For this review, take the finished solid that the model builds, in its own axes (mm). Face numbers are marked on the shaded views. A direction names the side the tool comes from. Coordinates: 2 decimals unless noted, no trailing zeros. Order: outer loops, then holes, each group sorted by start corner. A loop starts at its lowest first (then second) coordinate and runs counter-clockwise, first axis right, second up. Notation, with made-up numbers: (-12.5, 0.5) -> (41.5, 0.5) arc R30 cw to (41.5, 31.5) -> close; hole circle Ø9 at (-1.5, 63.25). An arc over 180 degrees is marked (long way). Answer as a JSON object with one key per item and string values. Group by question number.
1) For pin 1 (8 mm diameter, centred on x = -6, z = -4.5, fed in from -Y); pin 2 (2 mm diameter, centred on x = -7.5, y = 3, fed in from +Z); pin 3 (1 mm diameter, centred on x = -3.5, y = 3.5, fed in from +Z); pin 4 (5.5 mm diameter, centred on x = -10.5, z = 0, fed in from +Y), all flat-tipped, find the tip position at first contact; note any pin that passes through.
2) Add section C-C, the plane y = 0.7. Write out the cut boundary in (x, z), then the cut area to 3 significant figures.
3) Add section A-A, the plane x = -10.5. Write out the cut boundary in (y, z), then the cut area to 3 significant figures.
4) Machinability: for the marked faces 4, 5 and 6, which of the approach directions +Z, -Z, +X, -X, +Y, -Y give a long, thin tool a straight path to every point of the face, cutting with its end or side? Answer none if there is none.
5) Add section D-D, the plane x = -5.25. Write out the cut boundary in (y, z).
6) Wall thickness on L1, parallel to X at y = 0.7, z = 0; L2, parallel to Z at x = -10.5, y = 0.85; L3, parallel to X at y = 0.45, z = -1.5: over which ranges is each line inside the solid? List them lowest first.
7) Draft analysis for pull direction X (two halves, no side actions). For the marked faces 1, 2 and 3, state which applies: +X half, -X half, draft (parallel to the pull), parting line (faces both ways), or undercut.
Autodesk Inventor part; units mm, degrees
ref_plane "YZ Plane" through (0, 0, 0) normal (1, 0, 0) x (0, 1, 0)
ref_plane "XZ Plane" through (0, 0, 0) normal (0, 1, 0) x (-1, 0, 0)
ref_plane "XY Plane" through (0, 0, 0) normal (0, 0, 1) x (1, 0, 0)
sketch "Szkic1" plane through (0, 0, 0) normal (0, 1, 0) x (-1, 0, 0)
  line L0 (-15, 8) -> (15, 8)
  line L1 (15, 8) -> (15, -8)
  line L2 (15, -8) -> (-15, -8)
  line L3 (-15, -8) -> (-15, 8)
  line L4 (-15, 8) -> (15, -8) construction
  line L5 (15, 8) -> (-15, -8) construction
  line L6 (-6, 6) -> (6, 6)
  line L7 (6, 6) -> (6, -6)
  line L8 (6, -6) -> (-6, -6)
  line L9 (-6, -6) -> (-6, 6)
  line L10 (-6, 6) -> (6, -6) construction
  line L11 (6, 6) -> (-6, -6) construction
  circle A0 centre (0, 0) radius 1.75
  dimension "d0" = 30
  dimension "d1" = 16
  dimension "d2" = 12
  dimension "d3" = 12
  dimension "d4" = 3.5
extrude "Wyciągnięcie proste1" add sketch "Szkic1" along normal blind 1.4 contours L0 L1 L2 L3 | L6 L7 L8 L9 | A0
extrude "Wyciągnięcie proste2" add sketch "Szkic1" along normal blind 1.6 contours L6 L7 L8 L9 | A0
extrude "Wyciągnięcie proste3" cut sketch "Szkic1" along normal blind 1 contours A0
chamfer "Faza1" distance 4 angle 45 4 edges at (15, 0.7, 8) (15, 0.7, -8) (-15, 0.7, 8) (-15, 0.7, -8)
offset faces "Rozmiar1" outward -0.5 faces at (-3.6667, 0.4667, 8) (-12.3333, 0.4667, 6.6667) (12.3333, 0.4667, 6.6667) (15, 0.4667, 1.3333) (13.6667, 0.4667, -5.3333) (3.6667, 0.4667, -8) (-13.6667, 0.4667, -5.3333) (-15, 0.4667, -1.3333)
sketch "Szkic2" plane through (0, 1.4, 0) normal (0, 1, 0) x (1, 0, 0)
  line L0 (-6, -6) -> (6, -6)
  line L1 (-6, 6) -> (6, 6)
  line L2 (-6, -6) -> (6, -6)
  line L3 (6, -6) -> (6, 6)
  line L4 (6, 6) -> (-6, 6)
  line L5 (-6, 6) -> (-6, -6)
  line L6 (0, 0) -> (-10.5, 0)
  line L7 (-10.5, 0) -> (10.5, 0)
  circle A0 centre (10.5, 0) radius 1.75
  circle A1 centre (-10.5, 0) radius 1.75
  dimension "d16" = 10.5
  dimension "d17" = 21
  dimension "d18" = 3.5
  dimension "d19" = 3.5
extrude "Wyciągnięcie proste4" cut sketch "Szkic2" against normal blind 10 contours A0 | A1
sketch "Szkic4" plane through (0, 1.6, 0) normal (0, 1, 0) x (1, 0, 0)
  line L0 (-4.2511, -3.84) -> (-4.2511, 0)
  line L1 (5.76, 0) -> (4.32, 0)
  line L2 (-2.3311, 0) -> (-2.3311, 3.84)
  line L3 (4.32, 0) -> (4.32, 3.84)
  line L4 (0, -5.76) -> (0, 5.76)
  line L5 (0, 5.76) -> (0, -5.76)
  line L6 (5.76, -5.76) -> (-5.76, -5.76)
  line L7 (-5.76, -5.76) -> (5.76, -5.76)
  line L8 (4.32, 3.84) -> (-2.3311, 0)
  line L9 (5.76, -5.76) -> (5.76, 5.76)
  line L10 (5.76, 5.76) -> (5.76, -5.76)
  line L11 (5.76, 0) -> (-5.76, 0)
  line L12 (5.76, 5.76) -> (-5.76, 5.76)
  line L13 (-5.76, 5.76) -> (5.76, 5.76)
  line L14 (5.76, 5.76) -> (-5.76, 5.76)
  circle A0 centre (0, 0) radius 5.76
  line L15 (-5.76, -5.76) -> (-5.76, 5.76)
  line L16 (-5.76, 5.76) -> (-5.76, -5.76)
  line L17 (-5.76, 5.76) -> (-5.76, -5.76)
  line L18 (4.32, 0) -> (4.32, -3.84)
  line L19 (4.32, -3.84) -> (-2.3311, 0)
  line L20 (-2.3311, 0) -> (-2.3311, -3.84)
  line L21 (-4.2511, 3.84) -> (-4.2511, 0)
  line L22 (-2.3311, -3.84) -> (-4.2511, -3.84)
  line L23 (-2.3311, 3.84) -> (-4.2511, 3.84)
  line L24 (6, -6) -> (-6, -6)
  line L25 (6, 6) -> (-6, 6)
  line L26 (5.76, -5.76) -> (-5.76, -5.76)
  line L27 (-5.76, -5.76) -> (-5.76, 5.76)
  line L28 (-5.76, 5.76) -> (5.76, 5.76)
  line L29 (5.76, 5.76) -> (5.76, -5.76)
  point P0 (-16.6045, -17.9068)
  point P1 (5.76, -5.76)
  point P2 (-5.76, -5.76)
  point P3 (4.32, 3.8099)
  point P4 (4.3023, 3.8298)
  point P5 (4.3023, -3.8298)
  point P6 (4.32, -3.8099)
extrude "Wyciągnięcie proste5" add sketch "Szkic4" along normal blind 3.5 contours L0 L11 L20 L22 | L21 L23 L2 L11 | L8 L4 L11 | L11 L4 L19 | L8 A0 L3 L11 L4 | L11 L18 A0 L19 L4
move faces "Przesuń1" translate (0, -1.75, 0) faces at (-0.0229, 1, 0.3868)
properties part number "guzik"
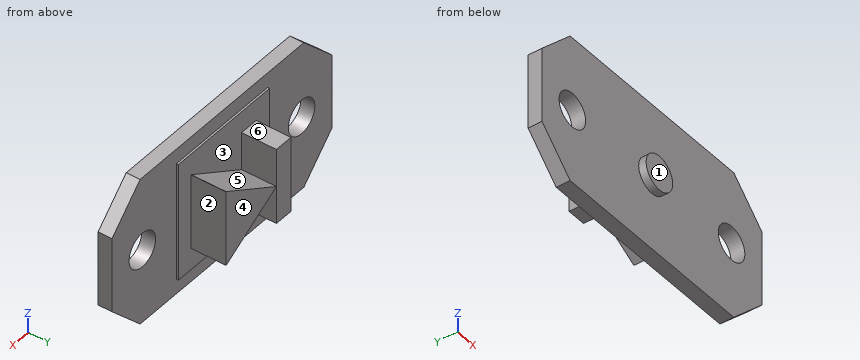
Output values:
{
 "1": {"pin 1": "stops at y = 0", "pin 2": "passes through", "pin 3": "stops at z = 3.84", "pin 4": "stops at y = 1.4"},
 "2": {"outline": "(-14.5, -3.79) -> (-10.79, -7.5) -> (10.79, -7.5) -> (14.5, -3.79) -> (14.5, 3.79) -> (10.79, 7.5) -> (-10.79, 7.5) -> (-14.5, 3.79) -> close; hole circle Ø3.5 at (-10.5, 0); hole circle Ø3.5 at (10.5, 0)", "area": "388 mm²"},
 "3": {"outline": "(0, -7.5) -> (1.4, -7.5) -> (1.4, -1.75) -> (0, -1.75) -> close; (0, 1.75) -> (1.4, 1.75) -> (1.4, 7.5) -> (0, 7.5) -> close", "area": "16.1 mm²"},
 "4": {"face 4": "+Z, -Z, +X, -X, +Y", "face 5": "+Z, +Y", "face 6": "+Z, +X, -X, +Y"},
 "5": {"outline": "(0, -7.5) -> (1.4, -7.5) -> (1.4, -6) -> (1.6, -6) -> (1.6, 6) -> (1.4, 6) -> (1.4, 7.5) -> (0, 7.5) -> close"},
 "6": {"L1": "x = -14.5 to -12.25, -8.75 to 8.75, 12.25 to 14.5", "L2": "z = -7.5 to -1.75, 1.75 to 7.5", "L3": "x = -14.5 to -11.4, -9.6 to 9.6, 11.4 to 14.5"},
 "7": {"face 1": "draft", "face 2": "+X half", "face 3": "undercut"}
}
